Autodesk Inventor part; units mm, degrees
ref_plane "YZ Plane" through (0, 0, 0) normal (1, 0, 0) x (0, 1, 0)
ref_plane "XZ Plane" through (0, 0, 0) normal (0, 1, 0) x (-1, 0, 0)
ref_plane "XY Plane" through (0, 0, 0) normal (0, 0, 1) x (1, 0, 0)
sketch "Sketch1" plane through (0, 0, 0) normal (1, 0, 0) x (0, 1, 0)
  line L0 (0.5, 107.169868) -> (0.5, -132.830132)
  line L1 (0.5, -132.830132) -> (5.5, -132.830132)
  line L2 (5.5, -132.830132) -> (5.5, -117.830132)
  line L3 (5.5, -117.830132) -> (6.5, -117.830132)
  line L4 (6.5, -117.830132) -> (6.5, -42.830132)
  line L5 (6.5, -42.830132) -> (6.5, -42.830132)
  line L6 (6.5, -42.830132) -> (6.5, 7.169868)
  line L7 (6.5, 7.169868) -> (6.5, 7.169868)
  line L8 (6.5, 7.169868) -> (6.5, 67.169868)
  line L9 (6.5, 67.169868) -> (5.5, 67.169868)
  line L10 (5.5, 67.169868) -> (5.5, 107.169868)
  line L11 (5.5, 107.169868) -> (0.5, 107.169868)
  circle A0 centre (0.5, 82.169868) radius 1.5
  point P0 (0, 0)
  dimension "d2" = 5
  dimension "d3" = 5
  dimension "d4" = 6
  dimension "d5" = 6
  dimension "d6" = 6
  dimension "d7" = 40
  dimension "d8" = 50
  dimension "d9" = 60
  dimension "d10" = 75
  dimension "d11" = 15
  dimension "d28" = 3
  dimension "d43" = 15
sketch "Sketch1 outline for Revolution2" plane through (0, 0, 0) normal (1, 0, 0) x (0, 1, 0)
  line L0 (5.5, 107.169868) -> (0.5, 107.169868)
  line L1 (5.5, 67.169868) -> (5.5, 107.169868)
  line L2 (6.5, 67.169868) -> (5.5, 67.169868)
  line L3 (6.5, 7.169868) -> (6.5, 67.169868)
  line L4 (6.5, -42.830132) -> (6.5, 7.169868)
  line L5 (6.5, -117.830132) -> (6.5, -42.830132)
  line L6 (5.5, -117.830132) -> (6.5, -117.830132)
  line L7 (5.5, -132.830132) -> (5.5, -117.830132)
  line L8 (0.5, -132.830132) -> (5.5, -132.830132)
  line L9 (0.5, 107.169868) -> (0.5, -132.830132)
revolve "Revolution2" add sketch "Sketch1 outline for Revolution2" angle 360 about axis through (0, 0.5, 107.169868) along (0, 0, -1)
chamfer "Chamfer1" distance 1 angle 45 6 edges at (0, -4.5, 107.1699) (0, -5.5, 67.1699) (0, -5.5, 7.1699) (0, -5.5, -42.8301) (0, -5.5, -117.8301) (0, -4.5, -132.8301)
thread "Thread2"
thread "Thread3"
sketch "Sketch1 outline for Extrusion2" plane through (0, 0, 0) normal (1, 0, 0) x (0, 1, 0)
  circle A0 centre (0.5, 82.169868) radius 1.5
extrude "Extrusion2" cut sketch "Sketch1 outline for Extrusion2" along normal through all both and the other way through all
thread "Thread4"
sketch "Sketch2" plane through (0, 0.5, 107.169868) normal (0, 0, 1) x (1, 0, 0)
  circle A0 centre (0, 0) radius 4
  circle A1 centre (0, 0) radius 2.5
  point P0 (0, -0.5)
  dimension "d35" = 5
sketch "Sketch2 outline for Extrusion3" plane through (0, 0.5, 107.169868) normal (0, 0, 1) x (1, 0, 0)
  circle A0 centre (0, 0) radius 2.5
extrude "Extrusion3" cut sketch "Sketch2 outline for Extrusion3" against normal blind 20
chamfer "Chamfer2" distance 1 angle 45 1 edges at (-2.5, 0.5, 107.1699)
thread "Thread5"
equation "\"d6\" = d5"
equation "\"d10\" = NagyKerékSzélesege"
equation "\"ZártSzelvényFalVastagság\" = 1.5"
equation "\"ZártSzelvényBelsőÁtmérő\" = 12"
equation "\"ZártSzelvényKülsőÁtmérő\" = 15"
equation "\"CsapágyBelsőÁtmérő\" = 12"
equation "\"CsapágySzélesége\" = 8"
equation "\"CsapágyKülsőÁtmérő\" = 28"
equation "\"CsapágyHázBelsőÁtmérő\" = 26"
equation "\"CsapágyHázHoszza\" = 45"
equation "\"CsapágyHázKülsőÁtmérő\" = 32"
equation "\"NagyKerékSzélesege\" = 75"
properties part number "NagyTengely"
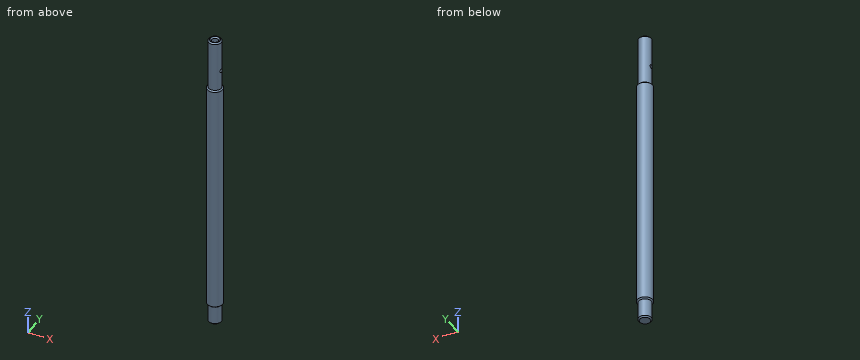
Geometry: final body of the model. Coordinates: model frame, mm. Round coordinates to 2 decimals unless told otherwise and drop trailing zeros. Loops run counter-clockwise (first coordinate to the right, second up) from the corner with the lowest first, then second, coordinate; pieces in that order, holes last.
Item 1: Contact query for flat-ended pins moving along their axis: P1, Ø6, axis at x = -4, z = -11, coming from the +Y side; P2, Ø1.5, axis at x = 1, z = -36, coming from the +Y side; P3, Ø5, axis at x = 2.5, z = 68, coming from the -Y side. Output: stop coordinate, or through.
Checked values:
P1: stops at y = 6.42
P2: stops at y = 6.49
P3: stops at y = -5.45
Item 2: Section B-B, the plane z = -58. Output: boundary loops of the cut face in (x, y).
Checked values:
outline: circle Ø12 at (0, 0.5)
Item 3: Line query: L1, parallel to Z at x = 0.5, y = 0.5; L2, parallel to Z at x = 4, y = 0.25; L3, parallel to X at y = 1, z = -54.5. Output: solid intervals per line, ascending.
Checked values:
L1: z = -132.83 to 80.67, 83.67 to 87.17
L2: z = -132.82 to 80.69, 83.65 to 107.16
L3: x = -5.98 to 5.98
